Source: CAD feature listing. Evaluate the final solid. Frame: model axes, mm. A direction names the side the tool comes from. Round coordinates to 2 decimals unless told otherwise and drop trailing zeros. Order: outer loops, then holes, each group sorted by start corner. A loop starts at its lowest first (then second) coordinate and runs counter-clockwise, first axis right, second up. Notation, with made-up numbers: M -8,61 L 37,61 A18 cw 37,95 Z; hole C 47,4 d6. An arc over 180 degrees is marked long. Answer as CSV lines item,"result". Start each with the question number.
Item 1: Section query C-C on x = -9.5. Return the cut outline in (y, z).
Item 2: Section query B-B on y = 10.5. Return the cut outline in (x, z), plus the area to 3 significant figures.
Item 3: Section query A-A on y = 0. Return the cut outline in (x, z), plus the area to 3 significant figures.
Item 4: Set-up query: faces 5 (the face through (-20.91, 6.75, 0.11)), 6 (the face through (-18, 12, 0)), 7 (the face through (24, -1, 0)). Return all of +Z, -Z, +X, -X, +Y, -Y with unobstructed straight access to the full face (end or side cutting, diameter ignored); none if empty.
Item 5: Pull-direction query (Z, two-part tool) for faces 1 (the face through (-17.5, 10, 0)), 2 (the face through (-29.5, -0.01, -6.07)), 3 (the face through (29.57, 0.01, 6)), 4 (the face through (27.75, 0.01, 0.08)); classes: +Z half, -Z half, draft (parallel to the pull), parting line (faces both ways), or undercut.
Item 6: Line query: line 1 (Z direction, x = 26, y = -0.1); line 2 (X direction, y = 11.5, z = 2.5); line 3 (X direction, y = 12.25, z = 1.25). Output: solid intervals per line, ascending. Write a range as [from, to].
Item 7: First-contact query: P1, Ø8, axis at y = 6.5, z = 3.5, coming from the -X side; P2, Ø1.1, axis at y = 11, z = -1, coming from the +X side; P3, Ø5, axis at x = 10, y = -2, coming from the -Z side; P4, Ø1.2, axis at x = 18, z = -3.5, coming from the -Y side. Flat tips, straight axial feed; report the tip coordinate or a pass-through.
Item 8: Section query D-D on z = 0. State how many separate pieces and enclosed holes the cut face has, plus the area to 3 significant figures.
from build123d import *

# Parameters (mm, degrees)
F1_DEPTH = 7.5
F3_DEPTH = 15
F4_R     = 1.75
F5_DEPTH = 25
F6_R     = 5


with BuildPart() as f1:
    # F0 (on Top) → F1 (new body, symmetric)
    with BuildSketch(Plane.XY):
        with BuildLine():
            ThreePointArc((-7, -8), (-15, 0), (-7, 8))
            Line((-7, 8), (7, 8))
            ThreePointArc((7, 8), (15, 0), (7, -8))
            Line((7, -8), (7, -9))
            Line((7, -9), (12, -9))
            ThreePointArc((12, -9), (15.5355339059, -7.5355339059), (17, -4))
            Line((17, -4), (17, -0.5764939444))
            ThreePointArc((17, -0.5764939444), (17.2314152463, 0.9270350531), (17.9042397786, 2.2913882374))
            Line((17.9042397786, 2.2913882374), (20.6383040886, 6.196036732))
            ThreePointArc((20.6383040886, 6.196036732), (20.9074339015, 6.7417780057), (21, 7.3431896047))
            Line((21, 7.3431896047), (21, 16))
            Line((21, 16), (17.5, 16))
            Line((17.5, 16), (17.5, 14))
            Line((17.5, 14), (19, 14))
            Line((19, 14), (19, 12))
            Line((19, 12), (17.5, 12))
            Line((17.5, 12), (17.5, 8.3))
            ThreePointArc((17.5, 8.3), (17.4540535831, 7.8737669717), (17.3183254055, 7.4671178237))
            ThreePointArc((17.3183254055, 7.4671178237), (16.5559000227, 7.003514385), (15.7267799625, 7.3333333333))
            ThreePointArc((15.7267799625, 7.3333333333), (14.0412414523, 8.5643546459), (12, 9))
            Line((12, 9), (-12, 9))
            ThreePointArc((-12, 9), (-14.0412414523, 8.5643546459), (-15.7267799625, 7.3333333333))
            ThreePointArc((-15.7267799625, 7.3333333333), (-16.5559000227, 7.003514385), (-17.3183254055, 7.4671178237))
            ThreePointArc((-17.3183254055, 7.4671178237), (-17.4540535831, 7.8737669717), (-17.5, 8.3))
            Line((-17.5, 8.3), (-17.5, 12))
            Line((-17.5, 12), (-19, 12))
            Line((-19, 12), (-19, 14))
            Line((-19, 14), (-17.5, 14))
            Line((-17.5, 14), (-17.5, 16))
            Line((-17.5, 16), (-21, 16))
            Line((-21, 16), (-21, 7.3431896047))
            ThreePointArc((-21, 7.3431896047), (-20.9074339015, 6.7417780057), (-20.6383040886, 6.196036732))
            Line((-20.6383040886, 6.196036732), (-17.9042397786, 2.2913882374))
            ThreePointArc((-17.9042397786, 2.2913882374), (-17.2314152463, 0.9270350531), (-17, -0.5764939444))
            Line((-17, -0.5764939444), (-17, -4))
            ThreePointArc((-17, -4), (-15.5355339059, -7.5355339059), (-12, -9))
            Line((-12, -9), (-7, -9))
            Line((-7, -9), (-7, -8))
        make_face()
    extrude(amount=F1_DEPTH, both=True)

    # F2 (on face) → F3 (join)
    with BuildSketch(Plane.XY.offset(7.5)):
        with BuildLine():
            Line((31, 1), (17.2550377406, 1))
            ThreePointArc((17.2550377406, 1), (17.0641712298, 0.2220011097), (17, -0.5764939444))
            Line((17, -0.5764939444), (17, -1))
            Line((17, -1), (31, -1))
            Line((31, -1), (31, 1))
        make_face()
        with BuildLine():
            Line((-31, -1), (-17, -1))
            Line((-17, -1), (-17, -0.5764939444))
            ThreePointArc((-17, -0.5764939444), (-17.0641712298, 0.2220011097), (-17.2550377406, 1))
            Line((-17.2550377406, 1), (-31, 1))
            Line((-31, 1), (-31, -1))
        make_face()
    extrude(amount=-F3_DEPTH)

    # F4 (on face) → F5 (cut)
    with BuildSketch(Plane(origin=(0, 1, 0), x_dir=(-1, 0, 0), z_dir=(0, 1, 0))):
        with Locations((-26, 0)):
            Circle(F4_R)
        with Locations((26, 0)):
            Circle(F4_R)
    extrude(amount=-F5_DEPTH, mode=Mode.SUBTRACT)

    # F6
    f6_edges = [f1.edges().sort_by_distance(p)[0] for p in [
        (-31, 0, -7.5),
        (-31, 0, 7.5),
        (31, 0, -7.5),
        (31, 0, 7.5),
    ]]
    fillet(f6_edges, radius=F6_R)


solid = f1.part
Results:
1,outline,"M -9,-7.5 L -7.6,-7.5 L -7.6,7.5 L -9,7.5 Z; M 7.6,-7.5 L 9,-7.5 L 9,7.5 L 7.6,7.5 Z"
2,outline,"M -21,-7.5 L -17.5,-7.5 L -17.5,7.5 L -21,7.5 Z; M 17.5,-7.5 L 21,-7.5 L 21,7.5 L 17.5,7.5 Z"
2,area,"105 mm^2"
3,outline,"M -31,-2.5 A5 ccw -26,-7.5 L -15,-7.5 L -15,7.5 L -26,7.5 A5 ccw -31,2.5 Z; M 15,-7.5 L 26,-7.5 A5 ccw 31,-2.5 L 31,2.5 A5 ccw 26,7.5 L 15,7.5 Z; hole C -26,0 d3.5; hole C 26,0 d3.5"
3,area,"439 mm^2"
4,face 5,"+Z, -Z, -X"
4,face 6,"+Z, -Z"
4,face 7,"+Z, -Z, +X, -Y"
5,face 1,"draft"
5,face 2,"-Z half"
5,face 3,"+Z half"
5,face 4,"undercut"
6,line 1,"[-7.5, -1.75], [1.75, 7.5]"
6,line 2,"[-21, -17.5], [17.5, 21]"
6,line 3,"[-21, -19], [19, 21]"
7,P1,"x = -21"
7,P2,"x = 21"
7,P3,"through"
7,P4,"y = -1"
8,separate pieces,"3"
8,enclosed holes,"0"
8,area,"278 mm^2"
